Geometry check sheet. Reference: the model listing, model coordinates, mm. A direction names the side the tool comes from. Round coordinates to 2 decimals unless told otherwise and drop trailing zeros. Loops run counter-clockwise (first coordinate to the right, second up) from the corner with the lowest first, then second, coordinate; pieces in that order, holes last. Notation, with made-up numbers: M -9.75,6.25 L 45.25,6.25 A28 cw 45.25,44.25 Z; hole C 53,89.25 d2. An arc over 180 degrees is marked long. Use one line per item in the form item = value. Start each with the question number.
1. Set-up check for faces 5 (the flat face through (6, -1, -15)), 6 (the flat face through (6, -1, 15)), 7 (the flat face through (-4, -1, -10)), 8 (the flat face through (-2.5, -1, 16)): record each of +Z, -Z, +X, -X, +Y, -Y from which the full face is reachable in a straight line by a thin tool's end or side.
2. Cross-section at B-B (x = 3). Record the boundary of the cut face in (y, z).
3. Cross-section at C-C (z = 7.5). Record the boundary of the cut face in (x, y), then the cut area to 4 significant figures.
4. Draft check along X on faces 1 (the flat face through (2.5, -1, 16)), 2 (the cylindrical face through (-3.5, -0.7, -14)), 3 (the cylindrical face through (3.5, -0.7, 14)), 4 (the flat face through (-1.5, -1, 0)). Enter one of: pulls with the +X half, pulls with the -X half, needs draft (parallel to the pull), parting line crosses it, or undercut.
5. Go/stop test with a flat-tipped pin: pin 1 (0.8 mm diameter, centred on y = -0.5, z = -16.5, fed in from -X). Record where the tip stops, or that it passes through.
6. Cross-section at A-A (y = -0.25). Record the boundary of the cut face in (x, z), then the cut area to 3 significant figures.
7. Material ranges on line 1 (Z direction, x = -4.75, y = -0.7); line 2 (Z direction, x = 3, y = -1.25); line 3 (X direction, y = -0.55, z = -8.5), recorded low to high.
```python
from build123d import *

# Parameters (mm, degrees)
F0_R     = 1.5
F1_DEPTH = 1.5


with BuildPart() as f1:
    # F0 (on Front) → F1 (new body)
    with BuildSketch(Plane.XZ):
        with BuildLine():
            Line((-4.5, 15), (-6, 15))
            Line((-6, 15), (-6, 11))
            ThreePointArc((-6, 11), (-5.707107, 10.292893), (-5, 10))
            Line((-5, 10), (-2.5, 10))
            ThreePointArc((-2.5, 10), (-1.792893, 9.707107), (-1.5, 9))
            Line((-1.5, 9), (-1.5, -9))
            ThreePointArc((-1.5, -9), (-1.792893, -9.707107), (-2.5, -10))
            Line((-2.5, -10), (-5, -10))
            ThreePointArc((-5, -10), (-5.707107, -10.292893), (-6, -11))
            Line((-6, -11), (-6, -15))
            Line((-6, -15), (-4.5, -15))
            ThreePointArc((-4.5, -15), (-3.5, -14), (-2.5, -15))
            Line((-2.5, -15), (-2.5, -17))
            Line((-2.5, -17), (2.5, -17))
            Line((2.5, -17), (2.5, -15))
            ThreePointArc((2.5, -15), (3.5, -14), (4.5, -15))
            Line((4.5, -15), (7, -15))
            Line((7, -15), (7, 15))
            Line((7, 15), (4.5, 15))
            ThreePointArc((4.5, 15), (3.5, 14), (2.5, 15))
            Line((2.5, 15), (2.5, 17))
            Line((2.5, 17), (-2.5, 17))
            Line((-2.5, 17), (-2.5, 15))
            ThreePointArc((-2.5, 15), (-3.5, 14), (-4.5, 15))
        make_face()
        with Locations((3, 0)):
            Circle(F0_R, mode=Mode.SUBTRACT)
    extrude(amount=F1_DEPTH)


solid = f1.part
```
Reported:
q1.face_5 = -Z, +X, +Y, -Y
q1.face_6 = +Z, +X, +Y, -Y
q1.face_7 = -X, +Y, -Y
q1.face_8 = +Z, -X, +Y, -Y
q2.outline = M -1.5,-14.13 L 0,-14.13 L 0,-1.5 L -1.5,-1.5 Z; M -1.5,1.5 L 0,1.5 L 0,14.13 L -1.5,14.13 Z
q3.outline = M -1.5,-1.5 L 7,-1.5 L 7,0 L -1.5,0 Z
q3.area = 12.75 mm²
q4.face_1 = pulls with the +X half
q4.face_2 = undercut
q4.face_3 = undercut
q4.face_4 = pulls with the -X half
q5.pin_1 = -2.5
q6.outline = M -6,-15 L -4.5,-15 A1 cw -2.5,-15 L -2.5,-17 L 2.5,-17 L 2.5,-15 A1 cw 4.5,-15 L 7,-15 L 7,15 L 4.5,15 A1 cw 2.5,15 L 2.5,17 L -2.5,17 L -2.5,15 A1 cw -4.5,15 L -6,15 L -6,11 A1 ccw -5,10 L -2.5,10 A1 cw -1.5,9 L -1.5,-9 A1 cw -2.5,-10 L -5,-10 A1 ccw -6,-11 Z; hole C 3,0 d3
q6.area = 307 mm²
q7.line_1 = -15 to -10, 10 to 15
q7.line_2 = -14.13 to -1.5, 1.5 to 14.13
q7.line_3 = -1.5 to 7
